Design review of the part built by this model. Coordinates are the model's own, in mm. A direction names the side the tool comes from. Coordinates: 2 decimals unless noted, no trailing zeros. Order: outer loops, then holes, each group sorted by start corner. A loop starts at its lowest first (then second) coordinate and runs counter-clockwise, first axis right, second up. Notation, with made-up numbers: (27.5, 46.5) -> (82.5, 46.5) arc R19 ccw to (82.5, 75.5) -> close; hole circle Ø6 at (52, 76). An arc over 180 degrees is marked (long way). Use a Markdown table: item, result. Add a question column.
Q1. Insertion check: pin 1 (1 mm diameter, centred on x = 9.5, y = 11, fed in from -Z); pin 2 (5 mm diameter, centred on x = 5, z = -7, fed in from +Y); pin 3 (7.5 mm diameter, centred on x = -2, z = 0.5, fed in from +Y). Each pin has a flat end and moves straight along its axis. Give the tip position at first contact, or say it passes through.
Q2. Add section B-B (x = 0). State the section outline as (y, z) points.
Q3. The part is to be moulded in two halves that separate along Z. For faces 4 (the face through (6.893, 13.303, 1.531)), 5 (the face through (0, -8, 0)), 6 (the face through (7.55, 7.71, -3.93)), say which applies: pulls with the +Z half, pulls with the -Z half, needs draft (parallel to the pull), parting line crosses it, or undercut.
Q4. Add section A-A (z = 10). Count the separate pieces of the cut face and the enclosed holes in it, then the cut area to 3 significant figures.
Q5. Add section C-C (y = -1). State the section outline as (x, z) points.
Q6. Add section D-D (z = 0). State the section outline as (x, y) points.
Q7. Wall thickness on probe 1 along Y at (x, z) = (-7.5, 5); probe 2 along Y at (x, z) = (9, 0.75); probe 3 along X at (y, z) = (7, 0): over which ranges is each line inside the solid? List them lowest first.
Q8. Machinability: for faces 1 (the face through (6.252, 13.667, -3.252)), 2 (the face through (0, 5.99, 0)), 3 (the face through (0, 0, 4)), which of the approach directions +Z, -Z, +X, -X, +Y, -Y give a long, thin tool a straight path to every point of the face, cutting with its end or side? Answer none if there is none.
from build123d import *

# Parameters (mm, degrees)
ESQUISSE2_R        = 3.3
BOSS_EXTRU_1_DEPTH = 8


with BuildPart() as part:
    # Esquisse1 → Révolution1 (revolve)
    with BuildSketch(Plane.XY, mode=Mode.PRIVATE) as r_volution1_sk:
        Polygon((0, 0), (8.227125787, 0), (8.227125787, 7.51998689), (12.727125787, 10.504949201), (8.227125787, 13.489911513), (12.727125787, 16.474873824), (12.284909149, 17.141540491), (6.779871333, 13.489911513), (11.279871333, 10.504949201), (7.427125787, 7.949326924), (7.427125787, 5.989911513), (0, 5.989911513), align=None)
    revolve(r_volution1_sk.sketch.rotate(Axis((0, 0, 0), (0, 1, 0)), 90), axis=Axis((0, 0, 0), (0, 1, 0)))

    # Esquisse2 → Boss.-Extru.1 (add)
    with BuildSketch(Plane.XZ):
        with Locations(Location((0, 0, 0), (0, 0, 270))):
            Circle(ESQUISSE2_R)
    extrude(amount=BOSS_EXTRU_1_DEPTH)


solid = part.part
Established:
| question | item | result |
|---|---|---|
| 1 | pin 1 | z = -8.61 |
| 1 | pin 2 | y = 16.36 |
| 1 | pin 3 | y = 5.99 |
| 2 | outline | (-8, -3.3) -> (0, -3.3) -> (0, -8.23) -> (7.52, -8.23) -> (10.5, -12.73) -> (13.49, -8.23) -> (16.47, -12.73) -> (17.14, -12.28) -> (13.49, -6.78) -> (10.5, -11.28) -> (7.95, -7.43) -> (5.99, -7.43) -> (5.99, 7.43) -> (7.95, 7.43) -> (10.5, 11.28) -> (13.49, 6.78) -> (17.14, 12.28) -> (16.47, 12.73) -> (13.49, 8.23) -> (10.5, 12.73) -> (7.52, 8.23) -> (0, 8.23) -> (0, 3.3) -> (-8, 3.3) -> close |
| 3 | face 4 | undercut |
| 3 | face 5 | needs draft |
| 3 | face 6 | parting line crosses it |
| 4 | separate pieces | 2 |
| 4 | enclosed holes | 1 |
| 4 | area | 39.8 mm^2 |
| 5 | outline | circle Ø6.6 at (0, 0) |
| 6 | outline | (-12.73, 10.5) -> (-8.23, 7.52) -> (-8.23, 0) -> (-3.3, 0) -> (-3.3, -8) -> (3.3, -8) -> (3.3, 0) -> (8.23, 0) -> (8.23, 7.52) -> (12.73, 10.5) -> (8.23, 13.49) -> (12.73, 16.47) -> (12.28, 17.14) -> (6.78, 13.49) -> (11.28, 10.5) -> (7.43, 7.95) -> (7.43, 5.99) -> (-7.43, 5.99) -> (-7.43, 7.95) -> (-11.28, 10.5) -> (-6.78, 13.49) -> (-12.28, 17.14) -> (-12.73, 16.47) -> (-8.23, 13.49) -> close |
| 7 | probe 1 | 8.04 to 9, 12.01 to 12.97, 14.01 to 14.97 |
| 7 | probe 2 | 8.05 to 9.01, 12 to 12.96, 14.02 to 14.98 |
| 7 | probe 3 | -8.23 to -7.43, 7.43 to 8.23 |
| 8 | face 1 | +Y |
| 8 | face 2 | none |
| 8 | face 3 | -Y |
